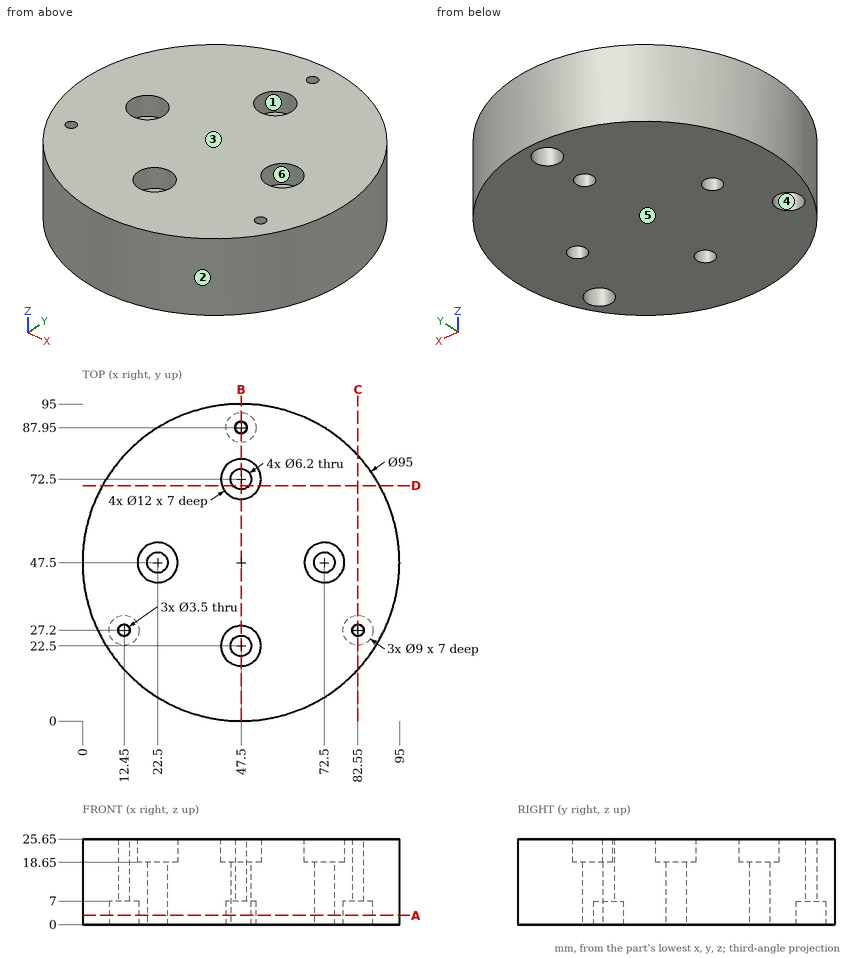
Drawing for the job (mm, zero at the part's lowest x, y, z). A direction names the side the tool comes from. Coordinates: 2 decimals unless noted, no trailing zeros. Write each loop counter-clockwise with the first axis right and the second up, starting at its lowest first coordinate (ties: lowest second). Pieces come first, ordered by that corner, then holes. Notation, with made-up numbers: (-26, 43) -> (14, 43) arc R27 cw to (14, 74) -> close; hole circle Ø3 at (-2.75, 5). An arc over 180 degrees is marked (long way). One line per item, written item: value. Start each with the question number.
1) Probe probe 1 along X at (y, z) = (26, 3.5); probe 2 along X at (y, z) = (28, 23.75); probe 3 along X at (y, z) = (45.5, 1.25). List the from-to ranges inside material, lowest first.
2) Pull direction Y, two halves, no side cores. Call the marked faces 1, 2 and 3: +Y half, -Y half, draft (parallel to the pull), parting line (faces both ways), or undercut.
3) Slice it at C-C on x = 82.55. Write the cut outline in (y, z).
4) Slice it at B-B on x = 47.5. Write the cut outline in (y, z).
5) Slice it at A-A on z = 2.75. Write the cut outline in (x, y), then the cut area to 3 significant figures.
6) Which spindle directions (+Z, -Z, +X, -X, +Y, -Y) get a long thin tool onto all of the face, cutting with end or side? Do the marked faces 4, 5 and 6. Say none if no direction does.
7) Flat gauge pins, fed straight in: pin 1 Ø1 at (y, z) = (14, 9) entering from -X; pin 2 Ø3 at (y, z) = (41, 22.5) entering from -X; pin 3 Ø9.5 at (x, y) = (48, 22) entering from +Z. Where does each tip first touch, or does it go through?
8) Slice it at D-D on y = 70.5. Write the cut outline in (x, z).
Answers follow:
1. probe 1: 5.14 to 8.11, 16.79 to 78.21, 86.89 to 89.86
1. probe 2: 4.19 to 10.89, 14.01 to 45.1, 49.9 to 80.99, 84.11 to 90.81
1. probe 3: 0.04 to 20.13, 24.87 to 70.13, 74.87 to 94.96
2. face 1: undercut
2. face 2: parting line
2. face 3: draft
3. outline: (15.44, 0) -> (22.7, 0) -> (22.7, 7) -> (25.45, 7) -> (25.45, 25.65) -> (15.44, 25.65) -> close; (28.95, 7) -> (31.7, 7) -> (31.7, 0) -> (79.56, 0) -> (79.56, 25.65) -> (28.95, 25.65) -> close
4. outline: (0, 0) -> (19.4, 0) -> (19.4, 18.65) -> (16.5, 18.65) -> (16.5, 25.65) -> (0, 25.65) -> close; (25.6, 0) -> (69.4, 0) -> (69.4, 18.65) -> (66.5, 18.65) -> (66.5, 25.65) -> (28.5, 25.65) -> (28.5, 18.65) -> (25.6, 18.65) -> close; (75.6, 0) -> (83.45, 0) -> (83.45, 7) -> (86.2, 7) -> (86.2, 25.65) -> (78.5, 25.65) -> (78.5, 18.65) -> (75.6, 18.65) -> close; (89.7, 7) -> (92.45, 7) -> (92.45, 0) -> (95, 0) -> (95, 25.65) -> (89.7, 25.65) -> close
5. outline: circle Ø95 at (47.5, 47.5); hole circle Ø9 at (12.45, 27.2); hole circle Ø6.2 at (22.5, 47.5); hole circle Ø9 at (47.5, 87.95); hole circle Ø6.2 at (47.5, 22.5); hole circle Ø6.2 at (47.5, 72.5); hole circle Ø6.2 at (72.5, 47.5); hole circle Ø9 at (82.55, 27.2)
5. area: 6,780 mm2
6. face 4: -Z
6. face 5: -Z, +X, -X, +Y, -Y
6. face 6: +Z
7. pin 1: x = 13.33
7. pin 2: x = 0.26
7. pin 3: z = 18.65
8. outline: (5.94, 0) -> (45.13, 0) -> (45.13, 18.65) -> (41.84, 18.65) -> (41.84, 25.65) -> (5.94, 25.65) -> close; (49.87, 0) -> (89.06, 0) -> (89.06, 25.65) -> (53.16, 25.65) -> (53.16, 18.65) -> (49.87, 18.65) -> close
